Design review of the part built by this model. Coordinates are the model's own, in mm. Round coordinates to 2 decimals unless told otherwise and drop trailing zeros. Write each loop counter-clockwise with the first axis right and the second up, starting at its lowest first coordinate (ties: lowest second). Pieces come first, ordered by that corner, then holes. Notation, with made-up numbers: (36.5, 42) -> (69.5, 42) arc R24 ccw to (69.5, 56) -> close; hole circle Ø5 at (46, 65). An arc over 180 degrees is marked (long way). One line per question, with ' | ' between items. Start each with the question number.
1) For probe 1 along Y at (x, z) = (0, 2); probe 2 along X at (y, z) = (-2.5, 1.8); probe 3 along X at (y, z) = (-6, 1.95), list the stretches that pass through material, from the lowest coordinate up.
2) Consider section C-C (x = 0). Give the boundary of the cut face in (y, z), then the cut area to 3 significant figures.
3) Consider section D-D (x = 25). Give the boundary of the cut face in (y, z), then the cut area to 3 significant figures.
4) Consider section A-A (y = 0). Give the boundary of the cut face in (x, z).
5) Consider section B-B (z = 2.35). Give the boundary of the cut face in (x, y), then the cut area to 3 significant figures.
6) Insertion check: pin 1 Ø1.5 at (x, z) = (13.5, 2.5) entering from +Y; pin 2 Ø1.5 at (y, z) = (-8.5, 1) entering from +X; pin 3 Ø10 at (x, y) = (0, 0) entering from +Z; pin 4 Ø3 at (x, y) = (0, -20) entering from +Z. Each pin has a flat end and moves straight along its axis. Give the tip position at first contact, or say it passes through.
```python
from build123d import *

# Parameters (mm, degrees)
CROQUIS1_R              = 3.05
CROQUIS1_R_2            = 1.75
SALIENTE_EXTRUIR1_DEPTH = 3


with BuildPart() as part:
    # Croquis1 → Saliente-Extruir1 (new body)
    with BuildSketch(Plane.XY):
        with BuildLine():
            Line((-36.932370625, 20), (-30.932370625, 20))
            Line((-30.932370625, 20), (-30.932370625, -20))
            Line((-30.932370625, -20), (-36.932370625, -20))
            Line((-36.932370625, -20), (-36.932370625, -25))
            Line((-36.932370625, -25), (-33.749074061, -25))
            ThreePointArc((-33.749074061, -25), (0, -42), (33.749074061, -25))
            Line((33.749074061, -25), (36.932370625, -25))
            Line((36.932370625, -25), (36.932370625, -20))
            Line((36.932370625, -20), (30.932370625, -20))
            Line((30.932370625, -20), (30.932370625, 20))
            Line((30.932370625, 20), (36.932370625, 20))
            Line((36.932370625, 20), (36.932370625, 25))
            Line((36.932370625, 25), (33.749074061, 25))
            ThreePointArc((33.749074061, 25), (0, 42), (-33.749074061, 25))
            Line((-33.749074061, 25), (-36.932370625, 25))
            Line((-36.932370625, 25), (-36.932370625, 20))
        make_face()
        Circle(CROQUIS1_R, mode=Mode.SUBTRACT)
        with Locations((0, 20)):
            Circle(CROQUIS1_R_2, mode=Mode.SUBTRACT)
        with Locations((0, -20)):
            Circle(CROQUIS1_R_2, mode=Mode.SUBTRACT)
    extrude(amount=SALIENTE_EXTRUIR1_DEPTH)


solid = part.part
```
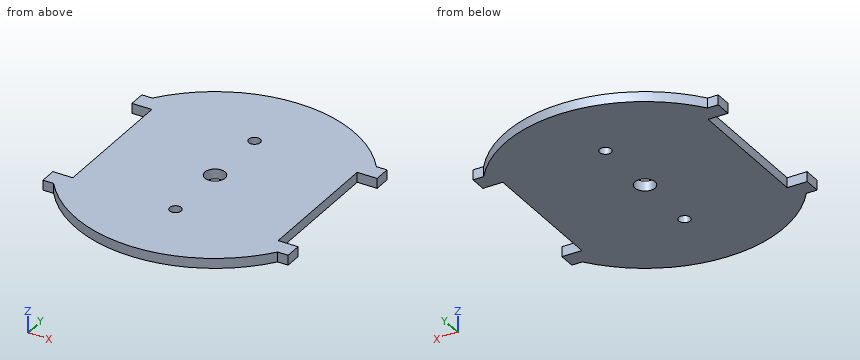
From the geometry:
1) probe 1: y = -42 to -21.75, -18.25 to -3.05, 3.05 to 18.25, 21.75 to 42 | probe 2: x = -30.93 to -1.75, 1.75 to 30.93 | probe 3: x = -30.93 to 30.93
2) outline: (-42, 0) -> (-21.75, 0) -> (-21.75, 3) -> (-42, 3) -> close; (-18.25, 0) -> (-3.05, 0) -> (-3.05, 3) -> (-18.25, 3) -> close; (3.05, 0) -> (18.25, 0) -> (18.25, 3) -> (3.05, 3) -> close; (21.75, 0) -> (42, 0) -> (42, 3) -> (21.75, 3) -> close | area: 213 mm2
3) outline: (-33.75, 0) -> (33.75, 0) -> (33.75, 3) -> (-33.75, 3) -> close | area: 202 mm2
4) outline: (-30.93, 0) -> (-3.05, 0) -> (-3.05, 3) -> (-30.93, 3) -> close; (3.05, 0) -> (30.93, 0) -> (30.93, 3) -> (3.05, 3) -> close
5) outline: (-36.93, -25) -> (-33.75, -25) arc R42 ccw to (33.75, -25) -> (36.93, -25) -> (36.93, -20) -> (30.93, -20) -> (30.93, 20) -> (36.93, 20) -> (36.93, 25) -> (33.75, 25) arc R42 ccw to (-33.75, 25) -> (-36.93, 25) -> (-36.93, 20) -> (-30.93, 20) -> (-30.93, -20) -> (-36.93, -20) -> close; hole circle Ø6.1 at (0, 0); hole circle Ø3.5 at (0, -20); hole circle Ø3.5 at (0, 20) | area: 4,770 mm2
6) pin 1: stops at y = 40.02 | pin 2: stops at x = 30.93 | pin 3: stops at z = 3 | pin 4: passes through
